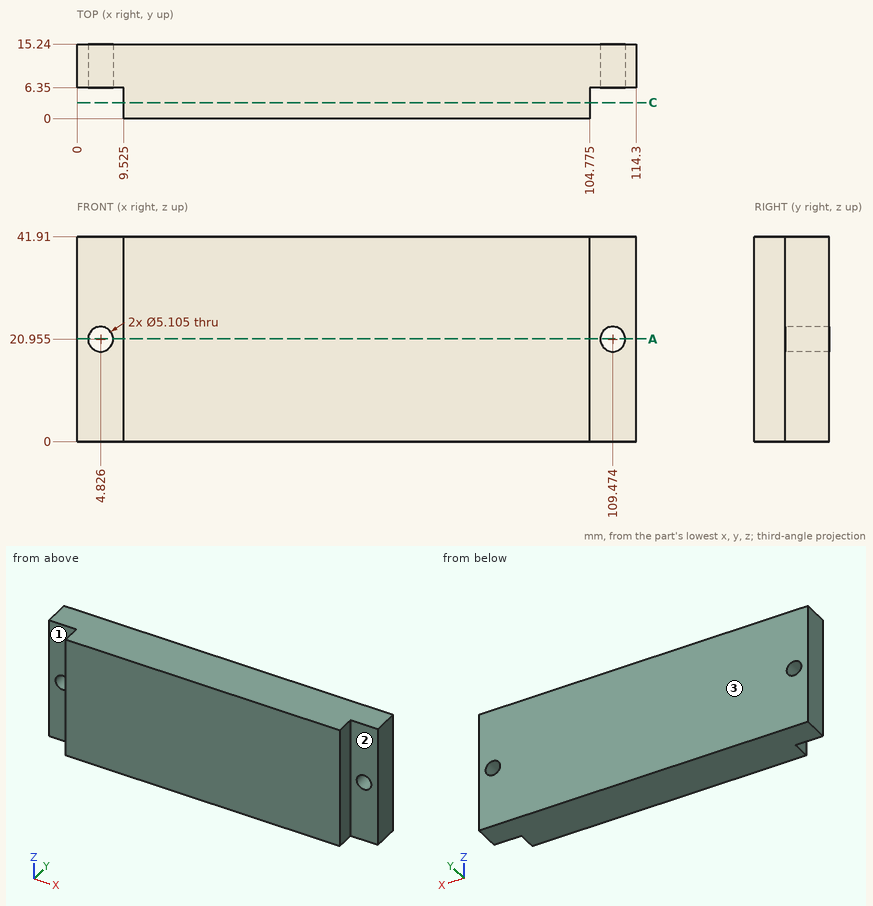
Answer from the drawing. Dimensions are ordinates in mm from the lowest x, y and z of the part. A direction names the side the tool comes from. Give positions to 0.01 mm unless a question says otherwise; leave off trailing zeros. Order: outer loops, then holes, each group sorted by start corner. A loop starts at its lowest first (then second) coordinate and runs counter-clockwise, first axis right, second up. Notation, with made-up numbers: (82.5, 43.5) - (90.5, 43.5) arc R17 ccw to (90.5, 52.5) - close; hole circle Ø1 at (15, -11). An arc over 180 degrees is marked (long way). Use one line per item in the form item = value.
1) For the marked faces 1, 2 and 3, determine the directions among +Z, -Z, +X, -X, +Y, -Y from which every point of the face is accessible in a straight line to the end or side of a thin tool.
Verdict:
face_1 = +Z, -Z, -X, -Y
face_2 = +Z, -Z, +X, -Y
face_3 = +Z, -Z, +X, -X, +Y
2) Find section C-C on y = 3.25. Determine the outline of the cut face in (x, z) (1 decimal).
Verdict:
outline = (9.5, 0) - (104.8, 0) - (104.8, 41.9) - (9.5, 41.9) - close
3) Consider probe 1 along Z at (x, y) = (5, 14.5); probe 2 along Y at (x, z) = (7.5, 6.5); probe 3 along X at (y, z) = (2, 28) (1 decimal). Determine where each line is inside the solid, lowest interval first. Write a range as [from, to].
Verdict:
probe_1 = [0, 18.41], [23.5, 41.91]
probe_2 = [6.35, 15.24]
probe_3 = [9.5, 104.8]
4) Each of these flat-tipped pins is pushed along its axis until it touches: pin 1 (5 mm diameter, centred on y = 2, z = 28, fed in from -X) (3 decimals); pin 2 (5 mm diameter, centred on x = 108, z = 31, fed in from -Y); pin 3 (1.9 mm diameter, centred on y = 3, z = 18.5, fed in from +X) (3 decimals); pin 4 (4.5 mm diameter, centred on x = 109.474, z = 20.955, fed in from +Y). Where does it stop, or does it pass through?
Verdict:
pin_1 = 9.525
pin_2 = 6.35
pin_3 = 104.775
pin_4 = through
5) Find section A-A on z = 21. Give the number of separate pieces and of enclosed holes in the cut face, and give its area (3 significant figures).
Verdict:
separate_pieces = 3
enclosed_holes = 0
area = 1,530 mm^2
